```python
from build123d import *

# Parameters (mm, degrees)
BOSS_EXTRU_2_DEPTH = 14.69
ESQUISSE2_W        = 9.88
ESQUISSE2_H        = 11.92
BOSS_EXTRU_3_DEPTH = 0.78
ESQUISSE3_R        = 1.655
BOSS_EXTRU_4_DEPTH = 7.17
ESQUISSE4_W        = 9.88
ESQUISSE4_H        = 11.92
BOSS_EXTRU_5_DEPTH = 0.78
ESQUISSE5_R        = 1.99
BOSS_EXTRU_6_DEPTH = 1.08


with BuildPart() as part:
    # Esquisse1 → Boss.-Extru.2 (new body)
    with BuildSketch(Plane.XY):
        with BuildLine():
            Line((0, 0), (0, 6.92))
            ThreePointArc((0, 6.92), (5.01, 9.47), (10.02, 6.92))
            Line((10.02, 6.92), (10.02, 0))
            ThreePointArc((10.02, 0), (5.01, -2.55), (0, 0))
        make_face()
    extrude(amount=BOSS_EXTRU_2_DEPTH)

    # Esquisse2 → Boss.-Extru.3 (add)
    with BuildSketch(Plane.XY.offset(14.69)):
        with Locations((5.01, 3.46)):
            Rectangle(ESQUISSE2_W, ESQUISSE2_H)
    extrude(amount=BOSS_EXTRU_3_DEPTH)

    # Esquisse3 → Boss.-Extru.4 (add)
    with BuildSketch(Plane.XY.offset(15.47)):
        with Locations((7.865, -0.125)):
            Circle(ESQUISSE3_R)
        with Locations((2.155, 7.045)):
            Circle(ESQUISSE3_R)
    extrude(amount=BOSS_EXTRU_4_DEPTH)

    # Esquisse4 → Boss.-Extru.5 (add)
    with BuildSketch(Plane.XY.offset(22.64)):
        with Locations((5.01, 3.46)):
            Rectangle(ESQUISSE4_W, ESQUISSE4_H)
    extrude(amount=BOSS_EXTRU_5_DEPTH)

    # Esquisse5 → Boss.-Extru.6 (add)
    with BuildSketch(Plane.XY.offset(23.42)):
        with Locations((5.01, 3.46)):
            Circle(ESQUISSE5_R)
    extrude(amount=BOSS_EXTRU_6_DEPTH)


solid = part.part
```
Part model, mm, in its own coordinate system. A direction names the side the tool comes from. Round coordinates to 2 decimals unless told otherwise and drop trailing zeros. Loops run counter-clockwise (first coordinate to the right, second up) from the corner with the lowest first, then second, coordinate; pieces in that order, holes last.
Item 1: Cut at D-D, the plane x = 9. Give the cut face in (y, z).
Item 2: Mould opens along Z. For faces 1 (the face through (2.7, 3.5, 23.42)), 2 (the face through (5, 4, 22.64)), 3 (the face through (4.93, 9.47, 7.24)) say: +Z half, -Z half, draft (parallel to the pull), parting line (faces both ways), or undercut.
Item 3: 3-axis set-ups, long thin cutter, end or side, ignore diameter. For faces 4 (the face through (5.09, -2.55, 7.24)), 5 (the face through (9, -2, 14.69)), 6 (the face through (1, 9, 14.69)), 7 (the face through (9, 9, 14.69)), 8 (the face through (1.8, 5.43, 19)): which of +Z, -Z, +X, -X, +Y, -Y reach the whole face in a straight line?
Item 4: Cut at A-A, the plane y = 3.46. Give the cut face in (x, z), then the cut area to 3 significant figures.
Item 5: Cut at B-B, the plane x = 5.01. Give the cut face in (y, z).
Item 6: Drill centre lines: line 1 (Z direction, x = 7.25, y = 7); line 2 (Z direction, x = 4, y = 4.5); line 3 (Y direction, x = 8, z = 2.5). Where is each one in solid material? Low to high.
Item 7: Drop flat-ended pins along their axis: P1, Ø0.9, axis at x = 3.5, z = 15, coming from the -Y side; P2, Ø0.6, axis at x = 3.5, z = 23, coming from the +Y side; P3, Ø0.9, axis at y = 2.5, z = 23, coming from the -X side. Give the stop position or say it passes through.
Item 8: Cut at C-C, the plane y = 0.5. Give the cut face in (x, z).
A:
1. outline: (-2.5, 14.69) - (-1.09, 14.69) - (-1.09, 0) - (8.01, 0) - (8.01, 14.69) - (9.42, 14.69) - (9.42, 15.47) - (1.08, 15.47) - (1.08, 22.64) - (9.42, 22.64) - (9.42, 23.42) - (-2.5, 23.42) - (-2.5, 22.64) - (-1.33, 22.64) - (-1.33, 15.47) - (-2.5, 15.47) - close
2. face 1: +Z half
2. face 2: undercut
2. face 3: draft
3. face 4: -Z, -Y
3. face 5: -Z, +X, -Y
3. face 6: -Z, -X, +Y
3. face 7: -Z, +X, +Y
3. face 8: none
4. outline: (0, 0) - (10.02, 0) - (10.02, 14.69) - (9.95, 14.69) - (9.95, 15.47) - (0.07, 15.47) - (0.07, 14.69) - (0, 14.69) - close; (0.07, 22.64) - (9.95, 22.64) - (9.95, 23.42) - (7, 23.42) - (7, 24.5) - (3.02, 24.5) - (3.02, 23.42) - (0.07, 23.42) - close
4. area: 167 mm2
5. outline: (-2.55, 0) - (9.47, 0) - (9.47, 14.69) - (9.42, 14.69) - (9.42, 15.47) - (-2.5, 15.47) - (-2.5, 14.69) - (-2.55, 14.69) - close; (-2.5, 22.64) - (9.42, 22.64) - (9.42, 23.42) - (5.45, 23.42) - (5.45, 24.5) - (1.47, 24.5) - (1.47, 23.42) - (-2.5, 23.42) - close
6. line 1: z = 0 to 15.47, 22.64 to 23.42
6. line 2: z = 0 to 15.47, 22.64 to 24.5
6. line 3: y = -1.78 to 8.7
7. P1: stops at y = -2.5
7. P2: stops at y = 9.42
7. P3: stops at x = 0.07
8. outline: (0, 0) - (10.02, 0) - (10.02, 14.69) - (9.95, 14.69) - (9.95, 15.47) - (9.4, 15.47) - (9.4, 22.64) - (9.95, 22.64) - (9.95, 23.42) - (0.07, 23.42) - (0.07, 22.64) - (6.33, 22.64) - (6.33, 15.47) - (0.07, 15.47) - (0.07, 14.69) - (0, 14.69) - close
